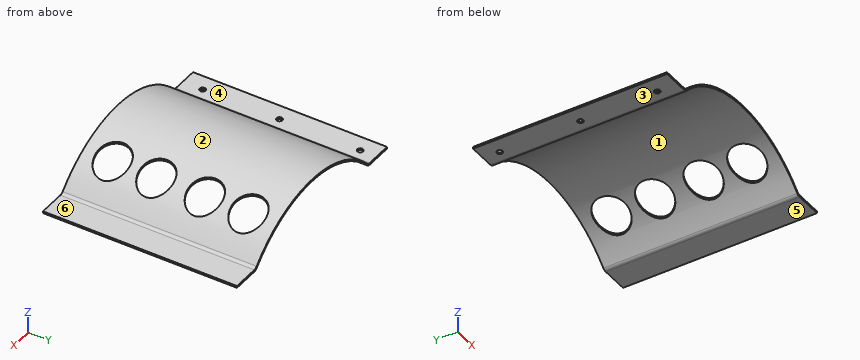
from build123d import *

# Parameters (mm, degrees)
F0_W     = 30
F0_H     = 2
F1_DEPTH = 200
F2_R     = 3
F3_DEPTH = 25
F2_R_2   = 17.5
F4_DEPTH = 50
F5_R     = 5
F6_R     = 5


with BuildPart() as f1:
    # F0 (on Front) → F1 (new body)
    with BuildSketch(Plane.XZ):
        with Locations((-105, 1)):
            Rectangle(F0_W, F0_H)
        with BuildLine():
            Line((-90, 2), (-90, 0))
            ThreePointArc((-90, 0), (0, 40), (90, 0))
            Line((90, 0), (90, 2))
            ThreePointArc((90, 2), (0, 42), (-90, 2))
        make_face()
        with Locations((105, 1)):
            Rectangle(F0_W, F0_H)
    extrude(amount=F1_DEPTH)

    # F2 (on face) → F3 (cut)
    with BuildSketch(Plane.XY.offset(2)):
        with Locations((-103.241667, -16.80618)):
            Circle(F2_R)
        with Locations((-103.241667, -100)):
            Circle(F2_R)
        with Locations((-103.241667, -179.280475)):
            Circle(F2_R)
    extrude(amount=-F3_DEPTH, mode=Mode.SUBTRACT)

    # F2 (on face) → F4 (cut)
    with BuildSketch(Plane.XY.offset(2)):
        with Locations((55, -30)):
            Circle(F2_R_2)
        with Locations((55, -75)):
            Circle(F2_R_2)
        with Locations((55, -125)):
            Circle(F2_R_2)
        with Locations((55, -170)):
            Circle(F2_R_2)
    extrude(amount=F4_DEPTH, mode=Mode.SUBTRACT)

    # F5
    f5_edges = [f1.edges().sort_by_distance(p)[0] for p in [
        (-90, -100, 0),
        (-90, -100, 2),
    ]]
    fillet(f5_edges, radius=F5_R)

    # F6
    f6_edges = [f1.edges().sort_by_distance(p)[0] for p in [
        (90, -100, 2),
        (90, -100, 0),
    ]]
    fillet(f6_edges, radius=F6_R)


solid = f1.part
The model under review builds one solid part; all positions refer to its coordinate system, in mm. Face numbers are marked on the shaded views. A direction names the side the tool comes from. Coordinates: 2 decimals unless noted, no trailing zeros. Loops run counter-clockwise (first coordinate to the right, second up) from the corner with the lowest first, then second, coordinate; pieces in that order, holes last. Notation, with made-up numbers: M -20,5.5 L 4,5.5 A32 ccw 4,38.5 Z; hole C -10.5,-33.5 d8. An arc over 180 degrees is marked long. Put each result on its own line as item: value. Start each with the question number.
Q1. Clearance check with flat-ended pins moving along their axes: pin 1 (5 mm diameter, centred on x = -103.24, y = -100, fed in from -Z); pin 2 (2 mm diameter, centred on y = -150, z = 27, fed in from -X); pin 3 (1.5 mm diameter, centred on x = -60, y = -66, fed in from -Z); pin 4 (8 mm diameter, centred on x = -81.5, y = -72.5, fed in from -Z). State where each tip first meets the part, or that it passes through.
Q2. Add section B-B (x = 55). Write out the cut boundary in (y, z).
Q3. For the marked faces 4, 5 and 6, list the 3-axis set-ups (+Z, -Z, +X, -X, +Y, -Y) from which the entire face can be reached by the end or side of a thin tool; tool diameter is ignored.
Q4. Add section C-C (z = 25). Write out the cut boundary in (x, y).
Q5. Wall thickness on line 1 (Z direction, x = 106.5, y = -122); line 2 (X direction, y = -55.5, z = 20.5); line 3 (X direction, y = -31, z = 8): over which ranges is each line inside the solid? List them lowest first.
Q6. Add section A-A (y = -100). Write out the cut boundary in (x, z), and give its area (3 significant figures).
Q7. Add section D-D (y = -52.5). Write out the cut boundary in (x, z).
Q8. The part is to be moulded in two halves that separate along X. For the marked faces 1, 2 and 3, say which applies: +X half, -X half, draft (parallel to the pull), parting line (faces both ways), or undercut.
Answers:
1. pin 1: passes through
1. pin 2: stops at x = -60.2
1. pin 3: stops at z = 23.68
1. pin 4: stops at z = 4.72
2. outline: M -200,26.81 L -187.5,26.81 L -187.5,28.81 L -200,28.81 Z; M -152.5,26.81 L -142.5,26.81 L -142.5,28.81 L -152.5,28.81 Z; M -107.5,26.81 L -92.5,26.81 L -92.5,28.81 L -107.5,28.81 Z; M -57.5,26.81 L -47.5,26.81 L -47.5,28.81 L -57.5,28.81 Z; M -12.5,26.81 L 0,26.81 L 0,28.81 L -12.5,28.81 Z
3. face 4: +Z, -X, +Y, -Y
3. face 5: -Z, +X, -X, +Y, -Y
3. face 6: +Z, +X, +Y, -Y
4. outline: M -61.92,-200 L -58.42,-200 L -58.42,0 L -61.92,0 Z; M 58.42,-200 L 61.92,-200 L 61.92,-186.08 A17.5 cw 58.42,-187.16 Z; M 58.42,-152.84 A17.5 cw 61.92,-153.92 L 61.92,-141.08 A17.5 cw 58.42,-142.16 Z; M 58.42,-107.84 A17.5 cw 61.92,-108.92 L 61.92,-91.08 A17.5 cw 58.42,-92.16 Z; M 58.42,-57.84 A17.5 cw 61.92,-58.92 L 61.92,-46.08 A17.5 cw 58.42,-47.16 Z; M 58.42,-12.84 A17.5 cw 61.92,-13.92 L 61.92,0 L 58.42,0 Z
5. line 1: z = 0 to 2
5. line 2: x = -68.93 to -65.94, 65.94 to 68.93
5. line 3: x = -84.2 to -82.07, 82.07 to 84.2
6. outline: M -120,0 L -106.24,0 L -106.24,2 L -120,2 Z; M -100.24,0 L -92.2,0 A5 ccw -88.54,1.58 A121.25 cw 88.54,1.58 A5 ccw 92.2,0 L 120,0 L 120,2 L 92.2,2 A5 cw 88.54,3.58 A121.25 ccw -88.54,3.58 A5 cw -92.2,2 L -100.24,2 Z
6. area: 468 mm^2
7. outline: M -120,0 L -92.2,0 A5 ccw -88.54,1.58 A121.25 cw 88.54,1.58 A5 ccw 92.2,0 L 120,0 L 120,2 L 92.2,2 A5 cw 88.54,3.58 A121.25 ccw -88.54,3.58 A5 cw -92.2,2 L -120,2 Z
8. face 1: undercut
8. face 2: parting line
8. face 3: draft
